Can you work these out from the model? Positions are in its coordinate system, mm. Face numbers are marked on the shaded views. Round coordinates to 2 decimals unless told otherwise and drop trailing zeros. Write each loop counter-clockwise with the first axis right and the second up, starting at its lowest first coordinate (ties: lowest second). Pieces come first, ordered by that corner, then holes.
Q1. We'd pull the mould along Z, two halves only. Please class the marked faces 1, 2 and 3: +Z half, -Z half, draft (parallel to the pull), parting line (faces both ways), or undercut.
Q2. If we section it at C-C (x = 82): Please give me the cut outline in (y, z).
Q3. If we section it at B-B (z = 32): Please give me the cut outline in (x, y).
Q4. Please list where these lines run through material, in increasing order: line 1 along X through (y, z) = (-7.5, 75.25); line 2 along X through (y, z) = (15, 73); line 3 along X through (y, z) = (7, 76).
Q5. If we section it at A-A (y = -15): Please give me the cut outline in (x, z), plus the area to 3 significant figures.
Q6. I'm going to push flat-ended pins straight in: pin 1 Ø5.5 at (y, z) = (25.42, 54.68) entering from +X; pin 2 Ø1.5 at (x, y) = (100.5, -15.5) entering from +Z. Where does each tip first touch, or does it pass through?
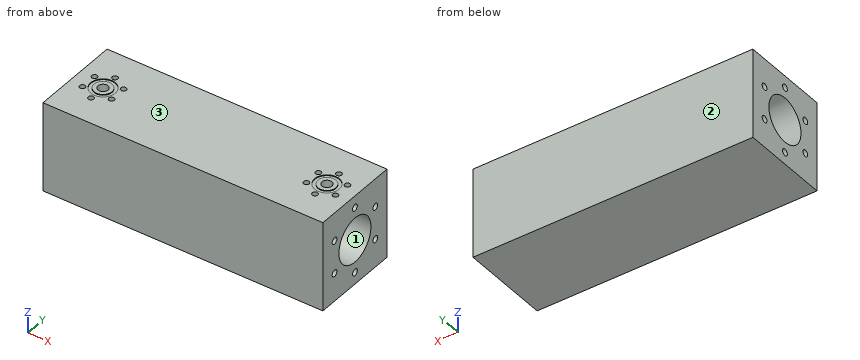
Solid Edge part; units mm, degrees
sketch "Sketch1" plane through (0, 0, 0) normal (0, 0, 1) x (1, 0, 0)
  line L0 (-125, -40) -> (125, -40)
  line L1 (125, -40) -> (125, 40)
  line L2 (125, 40) -> (-125, 40)
  line L3 (-125, 40) -> (-125, -40)
  dimension "D1" = 125
  dimension "D2" = 125
extrude "Protrusion1" add sketch "Sketch1" along normal blind 80
sketch "Sketch2" plane through (-125, 0, 75) normal (-1, 0, 0) x (0, -1, 0)
  circle A0 centre (0, -35) radius 20
extrude "Cutout1" cut sketch "Sketch2" against normal up to next
sketch "Sketch3" plane through (0, 0, 80) normal (0, 0, 1) x (0, -1, 0)
  circle A0 centre (0, -100) radius 4.5
  circle A1 centre (0, 100) radius 4.5
extrude "Cutout2" cut sketch "Sketch3" against normal up to next
hole "Hole_1" at (-100, 15, 80) direction (0, 0, -1) diameter 4.917 depth 12 thread major 6 thread length 10
pattern_circular "Pattern1" count 6 over 360 about axis through (-100, 0, 80) along (0, 0, -1) of "Hole_1"
sketch "Sketch4" plane through (0, 0, 80) normal (0, 0, 1) x (0, -1, 0)
  circle A0 centre (0, -100) radius 11
  circle A1 centre (0, -100) radius 8
extrude "CF16_groove" cut sketch "Sketch4" against normal blind 0.7
mirror "Mirror1" about plane through (0, 0, 0) normal (-1, 0, 0) of "Pattern1", "Hole_1", "CF16_groove"
hole "Hole_13" at (-125, 0, 10.65) direction (1, 0, 0) diameter 5.917 depth 20 thread major 7 thread length 18
pattern_circular "Pattern2" count 6 over 360 about axis through (-125, 0, 40) along (-1, 0, 0) of "Hole_13"
mirror "Mirror2" about plane through (0, 0, 0) normal (-1, 0, 0) of "Hole_13", "Pattern2"
A:
1. face 1: undercut
1. face 2: draft
1. face 3: +Z half
2. outline: (-40, 0) - (40, 0) - (40, 80) - (-40, 80) - close; hole circle Ø40 at (0, 40)
3. outline: (-125, -40) - (125, -40) - (125, -18.33) - (-125, -18.33) - close; (-125, 18.33) - (125, 18.33) - (125, 40) - (-125, 40) - close
4. line 1: x = -125 to -115.45, -110.53 to -89.47, -84.55 to 84.55, 89.47 to 110.53, 115.45 to 125
4. line 2: x = -125 to -102.46, -97.54 to 97.54, 102.46 to 125
4. line 3: x = -125 to -115.4, -110.58 to -89.42, -84.6 to 84.6, 89.42 to 110.58, 115.4 to 125
5. outline: (-125, 0) - (125, 0) - (125, 26.77) - (-125, 26.77) - close; (-125, 53.23) - (125, 53.23) - (125, 80) - (102.46, 80) - (102.46, 68) - (97.54, 68) - (97.54, 80) - (-97.54, 80) - (-97.54, 68) - (-102.46, 68) - (-102.46, 80) - (-125, 80) - close
5. area: 13,300 mm2
6. pin 1: stops at x = 105
6. pin 2: stops at z = 68
